```python
from build123d import *

# Parameters (mm, degrees)
SKETCH1_R           = 30.48
SKETCH1_R_2         = 2.15265
BOSS_EXTRUDE1_DEPTH = 2
CUT_EXTRUDE1_DEPTH  = 10


with BuildPart() as part:
    # Sketch1 → Boss-Extrude1 (new body)
    with BuildSketch(Plane(origin=(0, 0, 0), x_dir=(1, 0, 0), z_dir=(0, 1, 0))):
        with Locations(Location((0, 0, 0), (0, 0, 270))):
            Circle(SKETCH1_R)
        with Locations(Location((0, -23.8125, 0), (0, 0, 270))):
            Circle(SKETCH1_R_2, mode=Mode.SUBTRACT)
        with Locations(Location((20.622229928, -11.90625, 0), (0, 0, 270))):
            Circle(SKETCH1_R_2, mode=Mode.SUBTRACT)
        with Locations(Location((20.622229928, 11.90625, 0), (0, 0, 270))):
            Circle(SKETCH1_R_2, mode=Mode.SUBTRACT)
        with Locations(Location((0, 23.8125, 0), (0, 0, 270))):
            Circle(SKETCH1_R_2, mode=Mode.SUBTRACT)
        with Locations(Location((-20.622229928, 11.90625, 0), (0, 0, 270))):
            Circle(SKETCH1_R_2, mode=Mode.SUBTRACT)
        with Locations(Location((-20.622229928, -11.90625, 0), (0, 0, 270))):
            Circle(SKETCH1_R_2, mode=Mode.SUBTRACT)
    extrude(amount=BOSS_EXTRUDE1_DEPTH)

    # Sketch2 → Cut-Extrude1 (cut)
    with BuildSketch(Plane(origin=(0, 2, 0), x_dir=(1, 0, 0), z_dir=(0, 1, 0))):
        with BuildLine():
            ThreePointArc((1.93204455, 2.295038966), (-2.879237228, -0.842610814), (2.864533851, -0.8913169))
            Line((2.864533851, -0.8913169), (1.93204455, 2.295038966))
        make_face()
    extrude(amount=-CUT_EXTRUDE1_DEPTH, mode=Mode.SUBTRACT)


solid = part.part
```
Could you check a few things on this model? Use its own coordinates, in mm. A direction names the side the tool comes from. Round coordinates to 2 decimals unless told otherwise and drop trailing zeros. Write each loop counter-clockwise with the first axis right and the second up, starting at its lowest first coordinate (ties: lowest second). Pieces come first, ordered by that corner, then holes. Notation, with made-up numbers: M 56,1.25 L 81,1.25 A11 cw 81,11.25 Z; hole C -20,54.25 d8. An arc over 180 degrees is marked long. Answer in a Markdown table with one row per item. Add a question column.
Q1. Imagine slicing it at B-B (z = 0). Please give me the cut outline in (x, y), then the cut area to 3 significant figures.
Q2. If we mould it in two halves opening along Z, with no side actions, what happens to faces 1 (the cylindrical face through (30.22, 0.99, -3.97)), 2 (the cylindrical face through (-18.488, 0.986, 11.626)), 3 (the flat face through (-6, 2, 0))? For each: +Z half, -Z half, draft (parallel to the pull), parting line (faces both ways), or undercut.
Q3. Imagine slicing it at D-D (y = 1.7). Please give me the cut outline in (x, z).
Q4. If I drill on line 1 (X direction, y = 1.45, z = 10.5); line 2 (X direction, y = 0.85, z = -10); line 3 (X direction, y = 1.5, z = -22.5), over which ranges is the centre line in solid material (lowest first)? Write a range as from..to.
Q5. Will these pins go through, and if not, where does the flat tip stop? pin 1 Ø1 at (x, z) = (-22.5, 12) entering from -Y; pin 2 Ø1 at (x, y) = (-21.5, 1) entering from -Z.
Q6. Imagine slicing it at A-A (x = 0). Please give me the cut outline in (y, z).
Q7. Imagine slicing it at C-C (z = -12). Please give me the cut outline in (x, y).
Q8. On a 3-axis mill with a long thin cutter (end or side, diameter ignored), from which of +Z, -Z, +X, -X, +Y, -Y can I reach the whole of each face in a straight line? I mean faces 4 (the flat face through (2.4, 1, -0.7)), 5 (the flat face through (-6, 0, 0)). Say none if no direction works.
Values:
| question | item | result |
|---|---|---|
| 1 | outline | M -30.48,0 L -3,0 L -3,2 L -30.48,2 Z; M 2.6,0 L 30.48,0 L 30.48,2 L 2.6,2 Z |
| 1 | area | 111 mm^2 |
| 2 | face 1 | parting line |
| 2 | face 2 | undercut |
| 2 | face 3 | draft |
| 3 | outline | C 0,0 d60.96; hole C -20.62,-11.91 d4.31; hole C -20.62,11.91 d4.31; hole C 0,-23.81 d4.31; hole C 0,23.81 d4.31; hole M 1.93,-2.3 L 2.86,0.89 A3 ccw long Z; hole C 20.62,-11.91 d4.31; hole C 20.62,11.91 d4.31 |
| 4 | line 1 | -28.61..-22.25, -18.99..18.99, 22.25..28.61 |
| 4 | line 2 | -28.79..-21.62, -19.62..19.62, 21.62..28.79 |
| 4 | line 3 | -20.56..-1.71, 1.71..20.56 |
| 5 | pin 1 | y = 0 |
| 5 | pin 2 | z = -22.09 |
| 6 | outline | M 0,-30.48 L 2,-30.48 L 2,-25.97 L 0,-25.97 Z; M 0,-21.66 L 2,-21.66 L 2,-3 L 0,-3 Z; M 0,3 L 2,3 L 2,21.66 L 0,21.66 Z; M 0,25.97 L 2,25.97 L 2,30.48 L 0,30.48 Z |
| 7 | outline | M -28.02,0 L -22.77,0 L -22.77,2 L -28.02,2 Z; M -18.47,0 L 18.47,0 L 18.47,2 L -18.47,2 Z; M 22.77,0 L 28.02,0 L 28.02,2 L 22.77,2 Z |
| 8 | face 4 | +Y, -Y |
| 8 | face 5 | +Z, -Z, +X, -X, -Y |
